Check sheet for the modelled part. Datum: model origin and axes. Units: mm. Face numbers are marked on the shaded views. Round coordinates to 2 decimals unless told otherwise and drop trailing zeros. Loops run counter-clockwise (first coordinate to the right, second up) from the corner with the lowest first, then second, coordinate; pieces in that order, holes last. Notation, with made-up numbers: (24.5, -24.5) - (77.5, -24.5) arc R28 ccw to (77.5, 6.5) - close; hole circle Ø4 at (63, 86.5). An arc over 180 degrees is marked (long way). Put each result on its own line as item: value. Start each with the question number.
Item 1: Section check C-C, the plane z = -7.25. Record the cut outline in (x, y), and give its area (3 significant figures).
Item 2: Gauge pin test, flat ends, axial feed: pin 1 Ø8 at (y, z) = (-12, -0.5) entering from -X; pin 2 Ø1.5 at (x, z) = (-5.5, -7.5) entering from +Y; pin 3 Ø12 at (x, y) = (-13, 55.5) entering from +Z. Record the tip position at first contact, or that the pin passes through.
Item 3: Section check D-D, the plane x = 17. Record the cut outline in (y, z).
Item 4: Section check B-B, the plane y = -53. Record the cut outline in (x, z), and give its area (3 significant figures).
Item 5: Section check A-A, the plane x = 0. Record the cut outline in (y, z), and give its area (3 significant figures).
Item 6: Draft check along X on the marked faces 1 and 2. Enter one of: pulls with the +X half, pulls with the -X half, needs draft (parallel to the pull), parting line crosses it, or undercut.
Item 7: Material ranges on line 1 along X through (y, z) = (-42, -7); line 2 along Y through (x, z) = (0, 4); line 3 along Y through (x, z) = (-4, -7.25), recorded low to high.
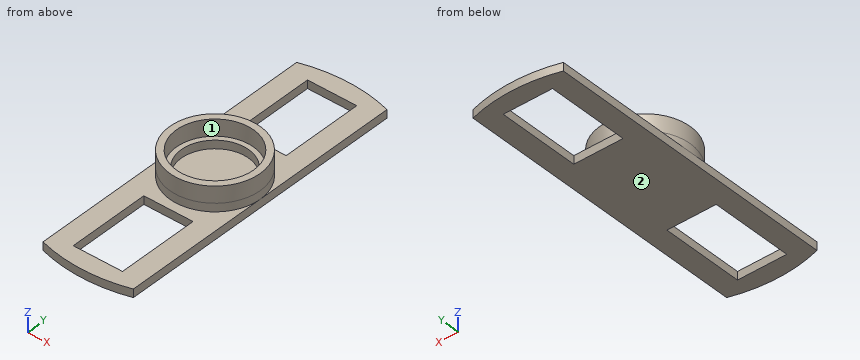
from build123d import *

# Parameters (mm, degrees)
SKETCH1_R           = 27.5
SKETCH1_R_2         = 23.5
BOSS_EXTRUDE1_DEPTH = 10
SKETCH2_R           = 27.5
SKETCH2_R_2         = 20.5
BOSS_EXTRUDE2_DEPTH = 5
BOSS_EXTRUDE3_DEPTH = 5
SKETCH4_W           = 30
SKETCH4_H           = 50
CUT_EXTRUDE1_DEPTH  = 10


with BuildPart() as part:
    # Sketch1 → Boss-Extrude1 (new body)
    with BuildSketch(Plane.XY):
        Circle(SKETCH1_R)
        Circle(SKETCH1_R_2, mode=Mode.SUBTRACT)
    extrude(amount=BOSS_EXTRUDE1_DEPTH)

    # Sketch2 → Boss-Extrude2 (add)
    with BuildSketch(Plane(origin=(0, 0, 0), x_dir=(-1, 0, 0), z_dir=(0, 0, -1))):
        Circle(SKETCH2_R)
        Circle(SKETCH2_R_2, mode=Mode.SUBTRACT)
    extrude(amount=BOSS_EXTRUDE2_DEPTH)

    # Sketch3 → Boss-Extrude3 (add)
    with BuildSketch(Plane(origin=(0, 0, -5), x_dir=(-1, 0, 0), z_dir=(0, 0, -1))):
        with BuildLine():
            Line((-27.5, 89.887429599), (-27.5, -89.887429599))
            ThreePointArc((-27.5, -89.887429599), (0, -94), (27.5, -89.887429599))
            Line((27.5, -89.887429599), (27.5, 89.887429599))
            ThreePointArc((27.5, 89.887429599), (0, 94), (-27.5, 89.887429599))
        make_face()
    extrude(amount=BOSS_EXTRUDE3_DEPTH)

    # Sketch4 → Cut-Extrude1 (cut)
    with BuildSketch(Plane.XY.offset(-5)):
        with Locations((0, -58)):
            Rectangle(SKETCH4_W, SKETCH4_H)
        with Locations((0, 58)):
            Rectangle(SKETCH4_W, SKETCH4_H)
    extrude(amount=-CUT_EXTRUDE1_DEPTH, mode=Mode.SUBTRACT)


solid = part.part
Check result:
1. outline: (-27.5, -89.89) arc R94 ccw to (27.5, -89.89) - (27.5, 89.89) arc R94 ccw to (-27.5, 89.89) - close; hole (-15, -83) - (15, -83) - (15, -33) - (-15, -33) - close; hole (-15, 33) - (15, 33) - (15, 83) - (-15, 83) - close
1. area: 7,190 mm²
2. pin 1: x = -26.31
2. pin 2: y = 93.88
2. pin 3: z = -5
3. outline: (-92.45, -10) - (92.45, -10) - (92.45, -5) - (21.62, -5) - (21.62, 10) - (16.22, 10) - (16.22, 0) - (11.46, 0) - (11.46, -5) - (-11.46, -5) - (-11.46, 0) - (-16.22, 0) - (-16.22, 10) - (-21.62, 10) - (-21.62, -5) - (-92.45, -5) - close
4. outline: (-27.5, -10) - (-15, -10) - (-15, -5) - (-27.5, -5) - close; (15, -10) - (27.5, -10) - (27.5, -5) - (15, -5) - close
4. area: 125 mm²
5. outline: (-94, -10) - (-83, -10) - (-83, -5) - (-94, -5) - close; (-33, -10) - (33, -10) - (33, -5) - (27.5, -5) - (27.5, 10) - (23.5, 10) - (23.5, 0) - (20.5, 0) - (20.5, -5) - (-20.5, -5) - (-20.5, 0) - (-23.5, 0) - (-23.5, 10) - (-27.5, 10) - (-27.5, -5) - (-33, -5) - close; (83, -10) - (94, -10) - (94, -5) - (83, -5) - close
5. area: 590 mm²
6. face 1: undercut
6. face 2: needs draft
7. line 1: -27.5 to -15, 15 to 27.5
7. line 2: -27.5 to -23.5, 23.5 to 27.5
7. line 3: -93.91 to -83, -33 to 33, 83 to 93.91
